Part print with two shaded views. Sizes in mm from the minimum x, y, z corner. A direction names the side the tool comes from. Coordinates: 2 decimals unless noted, no trailing zeros. Order: outer loops, then holes, each group sorted by start corner. A loop starts at its lowest first (then second) coordinate and runs counter-clockwise, first axis right, second up.
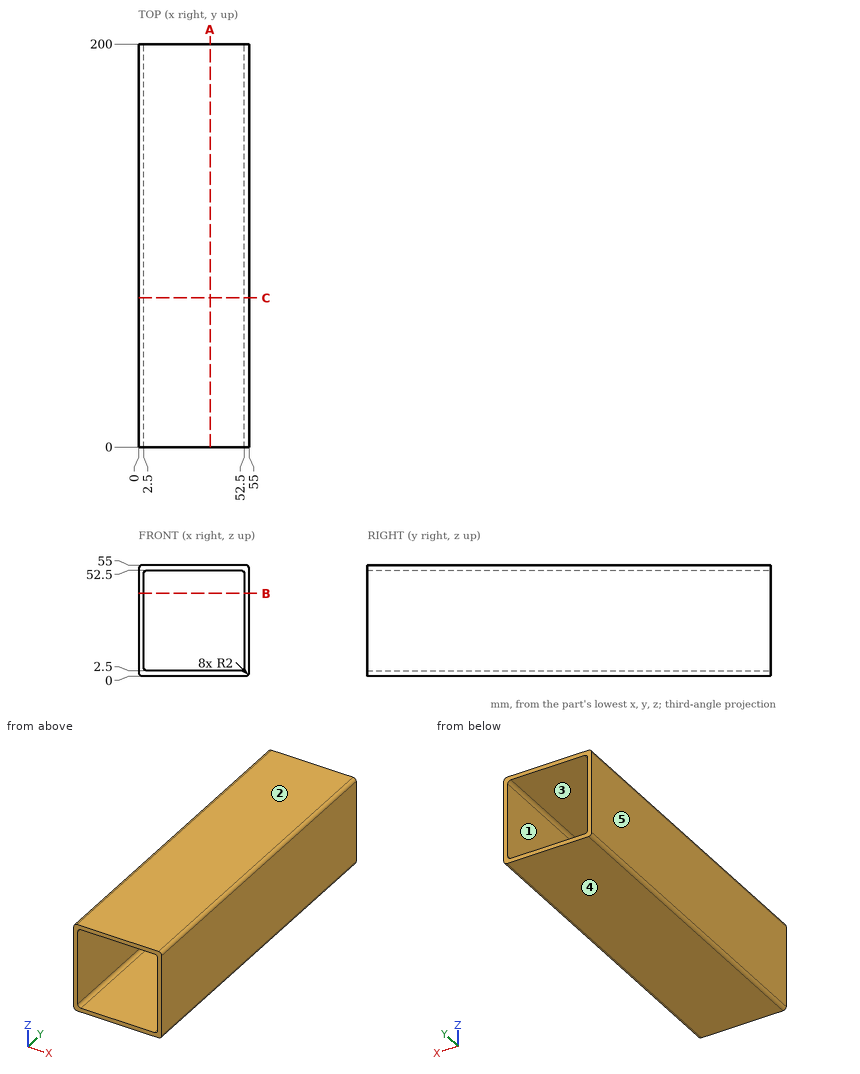
Q1. Wall check: line 1 along X through (y, z) = (17, 13); line 2 along X through (y, z) = (45, 3). Give the ranges that are in metal, low to high.
Results list:
line 1: x = 0 to 2.5, 52.5 to 55
line 2: x = 0 to 3.18, 51.82 to 55
Q2. Cut at B-B on z = 41. Write the cut outline in (x, y).
Results list:
outline: (0, 0) - (2.5, 0) - (2.5, 200) - (0, 200) - close; (52.5, 0) - (55, 0) - (55, 200) - (52.5, 200) - close
Q3. Cut at C-C on y = 74. Write the cut outline in (x, z), and give its area (3 significant figures).
Results list:
outline: (0, 2) arc R2 ccw to (2, 0) - (53, 0) arc R2 ccw to (55, 2) - (55, 53) arc R2 ccw to (53, 55) - (2, 55) arc R2 ccw to (0, 53) - close; hole (2.5, 4.5) arc R2 ccw to (4.5, 2.5) - (50.5, 2.5) arc R2 ccw to (52.5, 4.5) - (52.5, 50.5) arc R2 ccw to (50.5, 52.5) - (4.5, 52.5) arc R2 ccw to (2.5, 50.5) - close
area: 525 mm2
Q4. Pin check, flat tip, straight feed: pin 1 Ø5 at (x, z) = (5.5, 8.5) entering from -Y. Stop position of the tip, or through.
Results list:
pin 1: passes through
Q5. Mould opens along X. For the marked faces 3, 4 and 5 say: pulls with the +X half, pulls with the -X half, needs draft (parallel to the pull), parting line crosses it, or undercut.
Results list:
face 3: undercut
face 4: needs draft
face 5: pulls with the -X half
Q6. Cut at A-A on x = 35.5. Write the cut outline in (y, z).
Results list:
outline: (0, 0) - (200, 0) - (200, 2.5) - (0, 2.5) - close; (0, 52.5) - (200, 52.5) - (200, 55) - (0, 55) - close
Q7. Which spindle directions (+Z, -Z, +X, -X, +Y, -Y) get a long thin tool onto all of the face, cutting with end or side? Do the marked faces 1 and 2. Say none if no direction does.
Results list:
face 1: +Y, -Y
face 2: +Z, +X, -X, +Y, -Y
